Job drawing, mm, ordinate dimensions from the low corner. One solid piece. A direction names the side the tool comes from. Give positions to 0.01 mm unless a question says otherwise; leave off trailing zeros. Loops run counter-clockwise (first coordinate to the right, second up) from the corner with the lowest first, then second, coordinate; pieces in that order, holes last. Notation, with made-up numbers: (30, 62) - (81, 62) arc R18 ccw to (81, 73) - close; hole circle Ø7 at (56, 88). An arc over 180 degrees is marked (long way). Use a Markdown table: item, result.
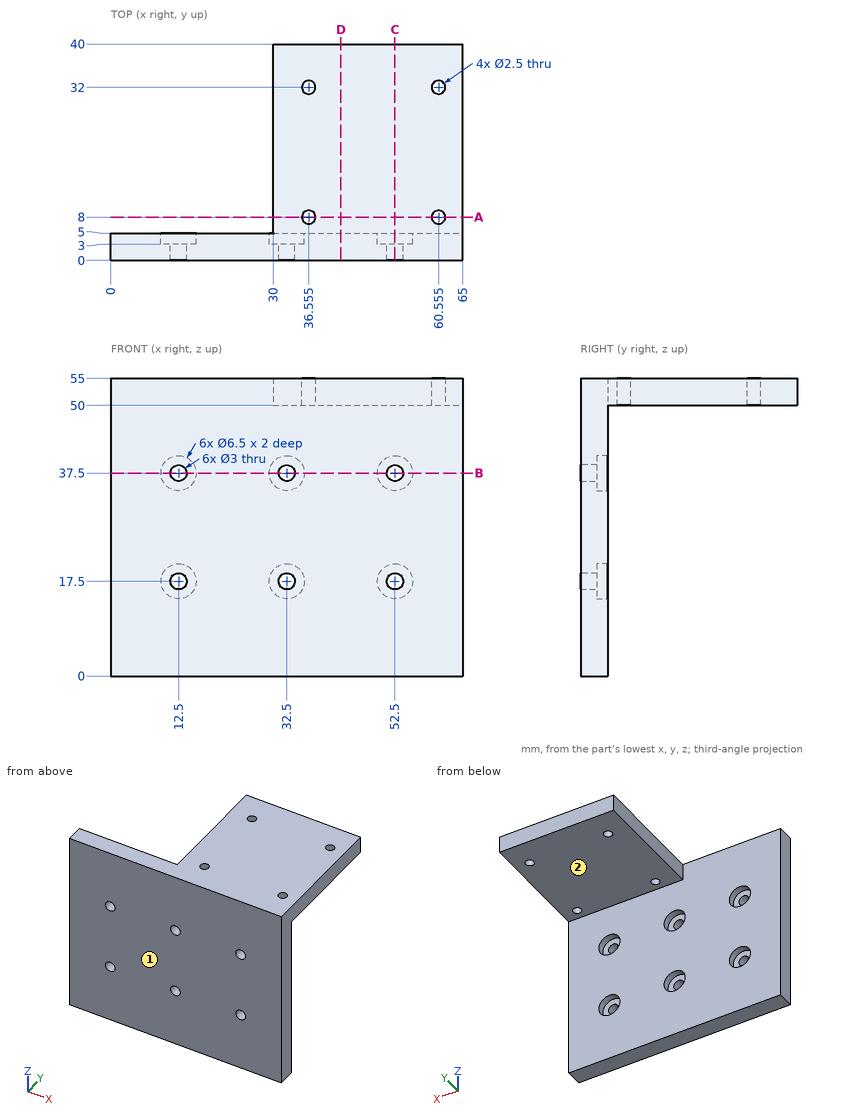
(1) Pin check, flat tips, straight feed: P1, Ø3, axis at x = 14, z = 37, coming from the +Y side; P2, Ø5, axis at x = 51, z = 38.5, coming from the +Y side; P3, Ø10.5, axis at x = 48, y = 18, coming from the -Z side. Stop position of each tip, or through.
Computed:
| item | result |
|---|---|
| P1 | y = 3 |
| P2 | y = 5 |
| P3 | z = 50 |
(2) 3-axis set-ups, long thin cutter, end or side, ignore diameter. For the marked faces 1 and 2: which of +Z, -Z, +X, -X, +Y, -Y reach the whole face in a straight line?
Computed:
| item | result |
|---|---|
| face 1 | +Z, -Z, +X, -X, -Y |
| face 2 | -Z, +X, -X, +Y |
(3) Slice it at A-A, the plane y = 8. Write the cut outline in (x, z) (1 decimal), plus the area to 3 significant figures.
Computed:
| item | result |
|---|---|
| outline | (30, 50) - (35.3, 50) - (35.3, 55) - (30, 55) - close; (37.8, 50) - (59.3, 50) - (59.3, 55) - (37.8, 55) - close; (61.8, 50) - (65, 50) - (65, 55) - (61.8, 55) - close |
| area | 150 mm² |
(4) Slice it at B-B, the plane z = 37.5. Write the cut outline in (x, y).
Computed:
| item | result |
|---|---|
| outline | (0, 0) - (11, 0) - (11, 3) - (9.25, 3) - (9.25, 5) - (0, 5) - close; (14, 0) - (31, 0) - (31, 3) - (29.25, 3) - (29.25, 5) - (15.75, 5) - (15.75, 3) - (14, 3) - close; (34, 0) - (51, 0) - (51, 3) - (49.25, 3) - (49.25, 5) - (35.75, 5) - (35.75, 3) - (34, 3) - close; (54, 0) - (65, 0) - (65, 5) - (55.75, 5) - (55.75, 3) - (54, 3) - close |
(5) Slice it at C-C, the plane x = 52.5. Write the cut outline in (y, z).
Computed:
| item | result |
|---|---|
| outline | (0, 0) - (5, 0) - (5, 14.25) - (3, 14.25) - (3, 16) - (0, 16) - close; (0, 19) - (3, 19) - (3, 20.75) - (5, 20.75) - (5, 34.25) - (3, 34.25) - (3, 36) - (0, 36) - close; (0, 39) - (3, 39) - (3, 40.75) - (5, 40.75) - (5, 50) - (40, 50) - (40, 55) - (0, 55) - close |
(6) Drill centre lines: probe 1 along X at (y, z) = (2.15, 17.5); probe 2 along Y at (x, z) = (4, 4.5); probe 3 along Z at (x, y) = (12, 3.5). Where is each one in solid material? Low to high. Write a range as [from, to].
Computed:
| item | result |
|---|---|
| probe 1 | [0, 11], [14, 31], [34, 51], [54, 65] |
| probe 2 | [0, 5] |
| probe 3 | [0, 14.29], [20.71, 34.29], [40.71, 55] |
(7) Slice it at D-D, the plane x = 42.5. Write the cut outline in (y, z), plus the area to 3 significant figures.
Computed:
| item | result |
|---|---|
| outline | (0, 0) - (5, 0) - (5, 50) - (40, 50) - (40, 55) - (0, 55) - close |
| area | 450 mm² |
